```python
from build123d import *

# Parameters (mm, degrees)
SKETCH_W  = 450
SKETCH_H  = 450
SKETCH_R  = 6.35
PAD_DEPTH = 6.35


with BuildPart() as part:
    # Sketch → Pad (new body)
    with BuildSketch(Plane.XY):
        with Locations((225, 225)):
            Rectangle(SKETCH_W, SKETCH_H)
        with Locations((67.471132, 382.456564)):
            Circle(SKETCH_R, mode=Mode.SUBTRACT)
        with Locations((102.47112, 382.485485)):
            Circle(SKETCH_R, mode=Mode.SUBTRACT)
        with Locations((137.471108, 382.514407)):
            Circle(SKETCH_R, mode=Mode.SUBTRACT)
        with Locations((172.471096, 382.543329)):
            Circle(SKETCH_R, mode=Mode.SUBTRACT)
        with Locations((207.471084, 382.57225)):
            Circle(SKETCH_R, mode=Mode.SUBTRACT)
        with Locations((242.471072, 382.601172)):
            Circle(SKETCH_R, mode=Mode.SUBTRACT)
        with Locations((277.47106, 382.630094)):
            Circle(SKETCH_R, mode=Mode.SUBTRACT)
        with Locations((312.471048, 382.659015)):
            Circle(SKETCH_R, mode=Mode.SUBTRACT)
        with Locations((347.471037, 382.687937)):
            Circle(SKETCH_R, mode=Mode.SUBTRACT)
        with Locations((382.471025, 382.716859)):
            Circle(SKETCH_R, mode=Mode.SUBTRACT)
        with Locations((67.500054, 347.456576)):
            Circle(SKETCH_R, mode=Mode.SUBTRACT)
        with Locations((102.500042, 347.485497)):
            Circle(SKETCH_R, mode=Mode.SUBTRACT)
        with Locations((137.50003, 347.514419)):
            Circle(SKETCH_R, mode=Mode.SUBTRACT)
        with Locations((172.500018, 347.543341)):
            Circle(SKETCH_R, mode=Mode.SUBTRACT)
        with Locations((207.500006, 347.572262)):
            Circle(SKETCH_R, mode=Mode.SUBTRACT)
        with Locations((242.499994, 347.601184)):
            Circle(SKETCH_R, mode=Mode.SUBTRACT)
        with Locations((277.499982, 347.630106)):
            Circle(SKETCH_R, mode=Mode.SUBTRACT)
        with Locations((312.49997, 347.659027)):
            Circle(SKETCH_R, mode=Mode.SUBTRACT)
        with Locations((347.499958, 347.687949)):
            Circle(SKETCH_R, mode=Mode.SUBTRACT)
        with Locations((382.499946, 347.716871)):
            Circle(SKETCH_R, mode=Mode.SUBTRACT)
        with Locations((67.528975, 312.456588)):
            Circle(SKETCH_R, mode=Mode.SUBTRACT)
        with Locations((102.528963, 312.485509)):
            Circle(SKETCH_R, mode=Mode.SUBTRACT)
        with Locations((137.528952, 312.514431)):
            Circle(SKETCH_R, mode=Mode.SUBTRACT)
        with Locations((172.52894, 312.543353)):
            Circle(SKETCH_R, mode=Mode.SUBTRACT)
        with Locations((207.528928, 312.572274)):
            Circle(SKETCH_R, mode=Mode.SUBTRACT)
        with Locations((242.528916, 312.601196)):
            Circle(SKETCH_R, mode=Mode.SUBTRACT)
        with Locations((277.528904, 312.630118)):
            Circle(SKETCH_R, mode=Mode.SUBTRACT)
        with Locations((312.528892, 312.659039)):
            Circle(SKETCH_R, mode=Mode.SUBTRACT)
        with Locations((347.52888, 312.687961)):
            Circle(SKETCH_R, mode=Mode.SUBTRACT)
        with Locations((382.528868, 312.716882)):
            Circle(SKETCH_R, mode=Mode.SUBTRACT)
        with Locations((67.557897, 277.4566)):
            Circle(SKETCH_R, mode=Mode.SUBTRACT)
        with Locations((102.557885, 277.485521)):
            Circle(SKETCH_R, mode=Mode.SUBTRACT)
        with Locations((137.557873, 277.514443)):
            Circle(SKETCH_R, mode=Mode.SUBTRACT)
        with Locations((172.557861, 277.543365)):
            Circle(SKETCH_R, mode=Mode.SUBTRACT)
        with Locations((207.557849, 277.572286)):
            Circle(SKETCH_R, mode=Mode.SUBTRACT)
        with Locations((242.557837, 277.601208)):
            Circle(SKETCH_R, mode=Mode.SUBTRACT)
        with Locations((277.557825, 277.630129)):
            Circle(SKETCH_R, mode=Mode.SUBTRACT)
        with Locations((312.557813, 277.659051)):
            Circle(SKETCH_R, mode=Mode.SUBTRACT)
        with Locations((347.557801, 277.687973)):
            Circle(SKETCH_R, mode=Mode.SUBTRACT)
        with Locations((382.55779, 277.716894)):
            Circle(SKETCH_R, mode=Mode.SUBTRACT)
        with Locations((67.586819, 242.456612)):
            Circle(SKETCH_R, mode=Mode.SUBTRACT)
        with Locations((102.586807, 242.485533)):
            Circle(SKETCH_R, mode=Mode.SUBTRACT)
        with Locations((137.586795, 242.514455)):
            Circle(SKETCH_R, mode=Mode.SUBTRACT)
        with Locations((172.586783, 242.543376)):
            Circle(SKETCH_R, mode=Mode.SUBTRACT)
        with Locations((207.586771, 242.572298)):
            Circle(SKETCH_R, mode=Mode.SUBTRACT)
        with Locations((242.586759, 242.60122)):
            Circle(SKETCH_R, mode=Mode.SUBTRACT)
        with Locations((277.586747, 242.630141)):
            Circle(SKETCH_R, mode=Mode.SUBTRACT)
        with Locations((312.586735, 242.659063)):
            Circle(SKETCH_R, mode=Mode.SUBTRACT)
        with Locations((347.586723, 242.687985)):
            Circle(SKETCH_R, mode=Mode.SUBTRACT)
        with Locations((382.586711, 242.716906)):
            Circle(SKETCH_R, mode=Mode.SUBTRACT)
        with Locations((67.61574, 207.456624)):
            Circle(SKETCH_R, mode=Mode.SUBTRACT)
        with Locations((102.615728, 207.485545)):
            Circle(SKETCH_R, mode=Mode.SUBTRACT)
        with Locations((137.615716, 207.514467)):
            Circle(SKETCH_R, mode=Mode.SUBTRACT)
        with Locations((172.615704, 207.543388)):
            Circle(SKETCH_R, mode=Mode.SUBTRACT)
        with Locations((207.615693, 207.57231)):
            Circle(SKETCH_R, mode=Mode.SUBTRACT)
        with Locations((242.615681, 207.601232)):
            Circle(SKETCH_R, mode=Mode.SUBTRACT)
        with Locations((277.615669, 207.630153)):
            Circle(SKETCH_R, mode=Mode.SUBTRACT)
        with Locations((312.615657, 207.659075)):
            Circle(SKETCH_R, mode=Mode.SUBTRACT)
        with Locations((347.615645, 207.687997)):
            Circle(SKETCH_R, mode=Mode.SUBTRACT)
        with Locations((382.615633, 207.716918)):
            Circle(SKETCH_R, mode=Mode.SUBTRACT)
        with Locations((67.644662, 172.456635)):
            Circle(SKETCH_R, mode=Mode.SUBTRACT)
        with Locations((102.64465, 172.485557)):
            Circle(SKETCH_R, mode=Mode.SUBTRACT)
        with Locations((137.644638, 172.514479)):
            Circle(SKETCH_R, mode=Mode.SUBTRACT)
        with Locations((172.644626, 172.5434)):
            Circle(SKETCH_R, mode=Mode.SUBTRACT)
        with Locations((207.644614, 172.572322)):
            Circle(SKETCH_R, mode=Mode.SUBTRACT)
        with Locations((242.644602, 172.601244)):
            Circle(SKETCH_R, mode=Mode.SUBTRACT)
        with Locations((277.64459, 172.630165)):
            Circle(SKETCH_R, mode=Mode.SUBTRACT)
        with Locations((312.644578, 172.659087)):
            Circle(SKETCH_R, mode=Mode.SUBTRACT)
        with Locations((347.644566, 172.688009)):
            Circle(SKETCH_R, mode=Mode.SUBTRACT)
        with Locations((382.644554, 172.71693)):
            Circle(SKETCH_R, mode=Mode.SUBTRACT)
        with Locations((67.673584, 137.456647)):
            Circle(SKETCH_R, mode=Mode.SUBTRACT)
        with Locations((102.673572, 137.485569)):
            Circle(SKETCH_R, mode=Mode.SUBTRACT)
        with Locations((137.67356, 137.514491)):
            Circle(SKETCH_R, mode=Mode.SUBTRACT)
        with Locations((172.673548, 137.543412)):
            Circle(SKETCH_R, mode=Mode.SUBTRACT)
        with Locations((207.673536, 137.572334)):
            Circle(SKETCH_R, mode=Mode.SUBTRACT)
        with Locations((242.673524, 137.601256)):
            Circle(SKETCH_R, mode=Mode.SUBTRACT)
        with Locations((277.673512, 137.630177)):
            Circle(SKETCH_R, mode=Mode.SUBTRACT)
        with Locations((312.6735, 137.659099)):
            Circle(SKETCH_R, mode=Mode.SUBTRACT)
        with Locations((347.673488, 137.688021)):
            Circle(SKETCH_R, mode=Mode.SUBTRACT)
        with Locations((382.673476, 137.716942)):
            Circle(SKETCH_R, mode=Mode.SUBTRACT)
        with Locations((67.702505, 102.456659)):
            Circle(SKETCH_R, mode=Mode.SUBTRACT)
        with Locations((102.702493, 102.485581)):
            Circle(SKETCH_R, mode=Mode.SUBTRACT)
        with Locations((137.702481, 102.514503)):
            Circle(SKETCH_R, mode=Mode.SUBTRACT)
        with Locations((172.702469, 102.543424)):
            Circle(SKETCH_R, mode=Mode.SUBTRACT)
        with Locations((207.702457, 102.572346)):
            Circle(SKETCH_R, mode=Mode.SUBTRACT)
        with Locations((242.702446, 102.601268)):
            Circle(SKETCH_R, mode=Mode.SUBTRACT)
        with Locations((277.702434, 102.630189)):
            Circle(SKETCH_R, mode=Mode.SUBTRACT)
        with Locations((312.702422, 102.659111)):
            Circle(SKETCH_R, mode=Mode.SUBTRACT)
        with Locations((347.70241, 102.688033)):
            Circle(SKETCH_R, mode=Mode.SUBTRACT)
        with Locations((382.702398, 102.716954)):
            Circle(SKETCH_R, mode=Mode.SUBTRACT)
        with Locations((67.731427, 67.456671)):
            Circle(SKETCH_R, mode=Mode.SUBTRACT)
        with Locations((102.731415, 67.485593)):
            Circle(SKETCH_R, mode=Mode.SUBTRACT)
        with Locations((137.731403, 67.514515)):
            Circle(SKETCH_R, mode=Mode.SUBTRACT)
        with Locations((172.731391, 67.543436)):
            Circle(SKETCH_R, mode=Mode.SUBTRACT)
        with Locations((207.731379, 67.572358)):
            Circle(SKETCH_R, mode=Mode.SUBTRACT)
        with Locations((242.731367, 67.60128)):
            Circle(SKETCH_R, mode=Mode.SUBTRACT)
        with Locations((277.731355, 67.630201)):
            Circle(SKETCH_R, mode=Mode.SUBTRACT)
        with Locations((312.731343, 67.659123)):
            Circle(SKETCH_R, mode=Mode.SUBTRACT)
        with Locations((347.731331, 67.688044)):
            Circle(SKETCH_R, mode=Mode.SUBTRACT)
        with Locations((382.731319, 67.716966)):
            Circle(SKETCH_R, mode=Mode.SUBTRACT)
    extrude(amount=PAD_DEPTH)


solid = part.part
```
Geometry check sheet. Reference: the model listing, model coordinates, mm. Round coordinates to 2 decimals unless told otherwise and drop trailing zeros. Use a Markdown table: item, result.
(1) Mould release check, pull along X, two halves, no side actions. Record for faces 1 (the cylindrical face through (342.993, 141.98, 3.131)), 2 (the cylindrical face through (136.73, 283.81, 3.13)): released by +X, released by -X, zero draft, split by the parting line, or undercut.
Calculated:
| item | result |
|---|---|
| face 1 | undercut |
| face 2 | undercut |
(2) Sectioned sample at A-A (z = 5). Give the number of separate pieces and of enclosed holes in the cut face, then the cut area to 3 significant figures.
Calculated:
| item | result |
|---|---|
| separate pieces | 1 |
| enclosed holes | 100 |
| area | 190,000 mm² |
(3) Go/stop test with a flat-tipped pin: P1, Ø11.5, axis at x = 172.47, y = 382.54, coming from the +Z side. Record where the tip stops, or that it passes through.
Calculated:
| item | result |
|---|---|
| P1 | through |
